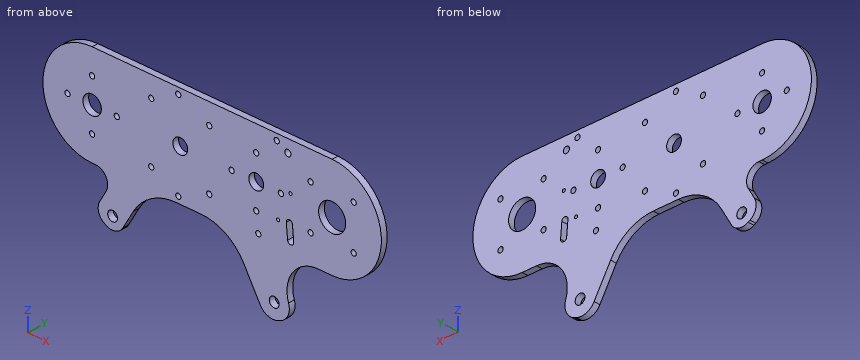
```python
from build123d import *

# Parameters (mm, degrees)
SKETCH1_R           = 11
SKETCH1_R_2         = 6
SKETCH1_R_3         = 7.5
SKETCH1_R_4         = 2.1
SKETCH1_R_5         = 2.5
SKETCH1_R_6         = 1.25
BOSS_EXTRUDE1_DEPTH = 5
SKETCH4_R           = 4
BOSS_EXTRUDE2_DEPTH = 5
FILLET1_R           = 40
FILLET2_R           = 10
CUT_EXTRUDE2_DEPTH  = 159.977801764
SKETCH7_R           = 4
BOSS_EXTRUDE3_DEPTH = 5
FILLET3_R           = 25
FILLET4_R           = 12
FILLET5_R           = 40


with BuildPart() as part:
    # Sketch1 → Boss-Extrude1 (new body)
    with BuildSketch(Plane(origin=(0, 0, 0), x_dir=(1, 0, 0), z_dir=(0, 1, 0))):
        with BuildLine():
            Line((-97.5, 40), (97.5, 40))
            ThreePointArc((97.5, 40), (137.5, 0), (97.5, -40))
            Line((97.5, -40), (-97.5, -40))
            ThreePointArc((-97.5, -40), (-137.5, 0), (-97.5, 40))
        make_face()
        with Locations(Location((97.5, 0, 0), (0, 0, 270))):
            Circle(SKETCH1_R, mode=Mode.SUBTRACT)
        with Locations(Location((35.8, 0, 0), (0, 0, 270))):
            Circle(SKETCH1_R_2, mode=Mode.SUBTRACT)
        with Locations(Location((-97.5, 0, 0), (0, 0, 270))):
            Circle(SKETCH1_R_3, mode=Mode.SUBTRACT)
        with Locations(Location((-97.5, -20, 0), (0, 0, 270))):
            Circle(SKETCH1_R_4, mode=Mode.SUBTRACT)
        with Locations(Location((-117.5, 0, 0), (0, 0, 270))):
            Circle(SKETCH1_R_4, mode=Mode.SUBTRACT)
        with Locations(Location((-97.5, 20, 0), (0, 0, 270))):
            Circle(SKETCH1_R_4, mode=Mode.SUBTRACT)
        with Locations(Location((-77.5, 0, 0), (0, 0, 270))):
            Circle(SKETCH1_R_4, mode=Mode.SUBTRACT)
        with Locations(Location((-25.9, 0, 0), (0, 0, 270))):
            Circle(SKETCH1_R_2, mode=Mode.SUBTRACT)
        with Locations(Location((-27.5, 35, 0), (0, 0, 270))):
            Circle(SKETCH1_R_4, mode=Mode.SUBTRACT)
        with Locations(Location((37.5, 35, 0), (0, 0, 270))):
            Circle(SKETCH1_R_4, mode=Mode.SUBTRACT)
        with Locations(Location((52.5, -35, 0), (0, 0, 270))):
            Circle(SKETCH1_R_4, mode=Mode.SUBTRACT)
        with Locations(Location((-27.5, -35, 0), (0, 0, 270))):
            Circle(SKETCH1_R_4, mode=Mode.SUBTRACT)
        with Locations(Location((115, 17.5, 0), (0, 0, 270))):
            Circle(SKETCH1_R_4, mode=Mode.SUBTRACT)
        with Locations(Location((115, -17.5, 0), (0, 0, 270))):
            Circle(SKETCH1_R_4, mode=Mode.SUBTRACT)
        with Locations(Location((80, -17.5, 0), (0, 0, 270))):
            Circle(SKETCH1_R_4, mode=Mode.SUBTRACT)
        with Locations(Location((80, 17.5, 0), (0, 0, 270))):
            Circle(SKETCH1_R_4, mode=Mode.SUBTRACT)
        with Locations(Location((55.8, 0, 0), (0, 0, 270))):
            Circle(SKETCH1_R_4, mode=Mode.SUBTRACT)
        with Locations(Location((35.8, -20, 0), (0, 0, 270))):
            Circle(SKETCH1_R_4, mode=Mode.SUBTRACT)
        with Locations(Location((15.8, 0, 0), (0, 0, 270))):
            Circle(SKETCH1_R_4, mode=Mode.SUBTRACT)
        with Locations(Location((35.8, 20, 0), (0, 0, 270))):
            Circle(SKETCH1_R_4, mode=Mode.SUBTRACT)
        with Locations(Location((-2.33, -23.57, 0), (0, 0, 270))):
            Circle(SKETCH1_R_4, mode=Mode.SUBTRACT)
        with Locations(Location((-49.47, -23.57, 0), (0, 0, 270))):
            Circle(SKETCH1_R_4, mode=Mode.SUBTRACT)
        with Locations(Location((-49.47, 23.57, 0), (0, 0, 270))):
            Circle(SKETCH1_R_4, mode=Mode.SUBTRACT)
        with Locations(Location((-2.33, 23.57, 0), (0, 0, 270))):
            Circle(SKETCH1_R_4, mode=Mode.SUBTRACT)
        with Locations(Location((61.5, -30, 0), (0, 0, 270))):
            Circle(SKETCH1_R_5, mode=Mode.SUBTRACT)
        with Locations(Location((53.643916542, 19.088290496, 0), (0, 0, 270))):
            Circle(SKETCH1_R_6, mode=Mode.SUBTRACT)
        with Locations(Location((63.643916542, -2.911709504, 0), (0, 0, 270))):
            Circle(SKETCH1_R_6, mode=Mode.SUBTRACT)
    extrude(amount=BOSS_EXTRUDE1_DEPTH)

    # Sketch4 → Boss-Extrude2 (add)
    with BuildSketch(Plane(origin=(0, 5, 0), x_dir=(1, 0, 0), z_dir=(0, 1, 0))):
        Polygon((-52.5, 40), (-77.5, 83.301270189), (-96.25, 72.475952642), (-77.5, 40), align=None)
        with Locations(Location((-80.857695155, 69.815698604, 0), (0, 0, 270))):
            Circle(SKETCH4_R, mode=Mode.SUBTRACT)
    extrude(amount=-BOSS_EXTRUDE2_DEPTH)

    # Fillet1
    fillet1_edges = [part.edges().sort_by_distance(p)[0] for p in [
        (-52.5, 2.5, -40),
    ]]
    fillet(fillet1_edges, radius=FILLET1_R)

    # Fillet2
    fillet2_edges = [part.edges().sort_by_distance(p)[0] for p in [
        (-77.5, 2.5, -40),
        (-96.25, 2.5, -72.475952642),
        (-77.5, 2.5, -83.301270189),
    ]]
    fillet(fillet2_edges, radius=FILLET2_R)

    # Sketch6 → Cut-Extrude2 (cut, through all)
    with BuildSketch(Plane(origin=(0, 5, 0), x_dir=(1, 0, 0), z_dir=(0, 1, 0))):
        with BuildLine():
            Line((65.244617832, 17.609884909), (66.290486745, 29.564221286))
            ThreePointArc((66.290486745, 29.564221286), (64.017889357, 32.272597388), (61.309513255, 30))
            Line((61.309513255, 30), (60.263644342, 18.045663623))
            ThreePointArc((60.263644342, 18.045663623), (62.53624173, 15.337287521), (65.244617832, 17.609884909))
        make_face()
    extrude(amount=-CUT_EXTRUDE2_DEPTH, mode=Mode.SUBTRACT)

    # Sketch7 → Boss-Extrude3 (add)
    with BuildSketch(Plane(origin=(0, 5, 0), x_dir=(1, 0, 0), z_dir=(0, 1, 0))):
        Polygon((14.047921201, 40), (42.5, 40), (67.5, 83.301270189), (44.047921201, 91.961524227), align=None)
        with Locations(Location((50.398774162, 76.961524227, 0), (0, 0, 270))):
            Circle(SKETCH7_R, mode=Mode.SUBTRACT)
    extrude(amount=-BOSS_EXTRUDE3_DEPTH)

    # Fillet3
    fillet3_edges = [part.edges().sort_by_distance(p)[0] for p in [
        (42.5, 2.5, -40),
    ]]
    fillet(fillet3_edges, radius=FILLET3_R)

    # Fillet4
    fillet4_edges = [part.edges().sort_by_distance(p)[0] for p in [
        (44.047921201, 2.5, -91.961524227),
        (67.5, 2.5, -83.301270189),
    ]]
    fillet(fillet4_edges, radius=FILLET4_R)

    # Fillet5
    fillet5_edges = [part.edges().sort_by_distance(p)[0] for p in [
        (14.047921201, 2.5, -40),
    ]]
    fillet(fillet5_edges, radius=FILLET5_R)


solid = part.part
```
Design review of the part built by this model. Coordinates are the model's own, in mm. Give positions to 0.01 mm unless a question says otherwise; leave off trailing zeros. Write each loop counter-clockwise with the first axis right and the second up, starting at its lowest first coordinate (ties: lowest second). Pieces come first, ordered by that corner, then holes. Notation, with made-up numbers: (17.5, -29) - (70.5, -29) arc R25 cw to (70.5, -12) - close; hole circle Ø9 at (0.5, 45.5). An arc over 180 degrees is marked (long way). Return JSON: item names as keys, results as strings. Group by question number.
(1) We need section D-D, the plane y = 2.6. Give the number of separate pieces and of enclosed holes in the cut face, then the cut area to 3 significant figures.
(2) Insertion check: pin 1 (1 mm diameter, centred on x = 70.5, y = 1.5, fed in from -Z); pin 2 (1 mm diameter, centred on y = 1, z = -30, fed in from +X); pin 3 (1 mm diameter, centred on y = 2.5, z = -62.5, fed in from -X). Each pin has a flat end and moves straight along its axis. Give the tip position at first contact, or say it passes through.
(3) We need section C-C, the plane x = 5. Give the boundary of the cut face in (y, z), then the cut area to 3 significant figures.
(4) We need section A-A, the plane z = 30. Give the boundary of the cut face in (x, y).
(5) To check wall thickness, follow probe 1 along Z at (x, y) = (35, 4.2); probe 2 along X at (y, z) = (2.25, 23.57); probe 3 along X at (y, z) = (2.8, -67.5). State the ranges of each line that lie inside material, in increasing order.
(6) We need section B-B, the plane z = -43.5. Give the boundary of the cut face in (x, y), then the cut area to 3 significant figures.
Reported:
{
 "1": {"separate pieces": "1", "enclosed holes": "30", "area": "22,200 mm2"},
 "2": {"pin 1": "stops at z = -45.63", "pin 2": "stops at x = 124.51", "pin 3": "stops at x = -90.78"},
 "3": {"outline": "(0, -42.55) - (5, -42.55) - (5, 40) - (0, 40) - close", "area": "413 mm2"},
 "4": {"outline": "(-123.96, 0) - (59, 0) - (59, 5) - (-123.96, 5) - close; (64, 0) - (123.96, 0) - (123.96, 5) - (64, 5) - close"},
 "5": {"probe 1": "z = -76.29 to -21.94, -18.06 to -5.95, 5.95 to 18.06, 21.94 to 40", "probe 2": "x = -129.82 to -51.57, -47.37 to -4.43, -0.23 to 129.82", "probe 3": "x = -92.5 to -84.12, -77.6 to -68.38, 29.93 to 60.93"},
 "6": {"outline": "(-87.22, 0) - (-45.77, 0) - (-45.77, 5) - (-87.22, 5) - close; (7.32, 0) - (73.04, 0) - (73.04, 5) - (7.32, 5) - close", "area": "536 mm2"}
}
